Part print with two shaded views. Sizes in mm from the minimum x, y, z corner. Give positions to 0.01 mm unless a question says otherwise; leave off trailing zeros. Order: outer loops, then holes, each group sorted by start corner. A loop starts at its lowest first (then second) coordinate and runs counter-clockwise, first axis right, second up. Notation, with made-up numbers: M 66.25,76 L 87.25,76 A24 cw 87.25,95 Z; hole C 35,48 d8. An arc over 180 degrees is marked long. Answer as CSV lines item,"result".
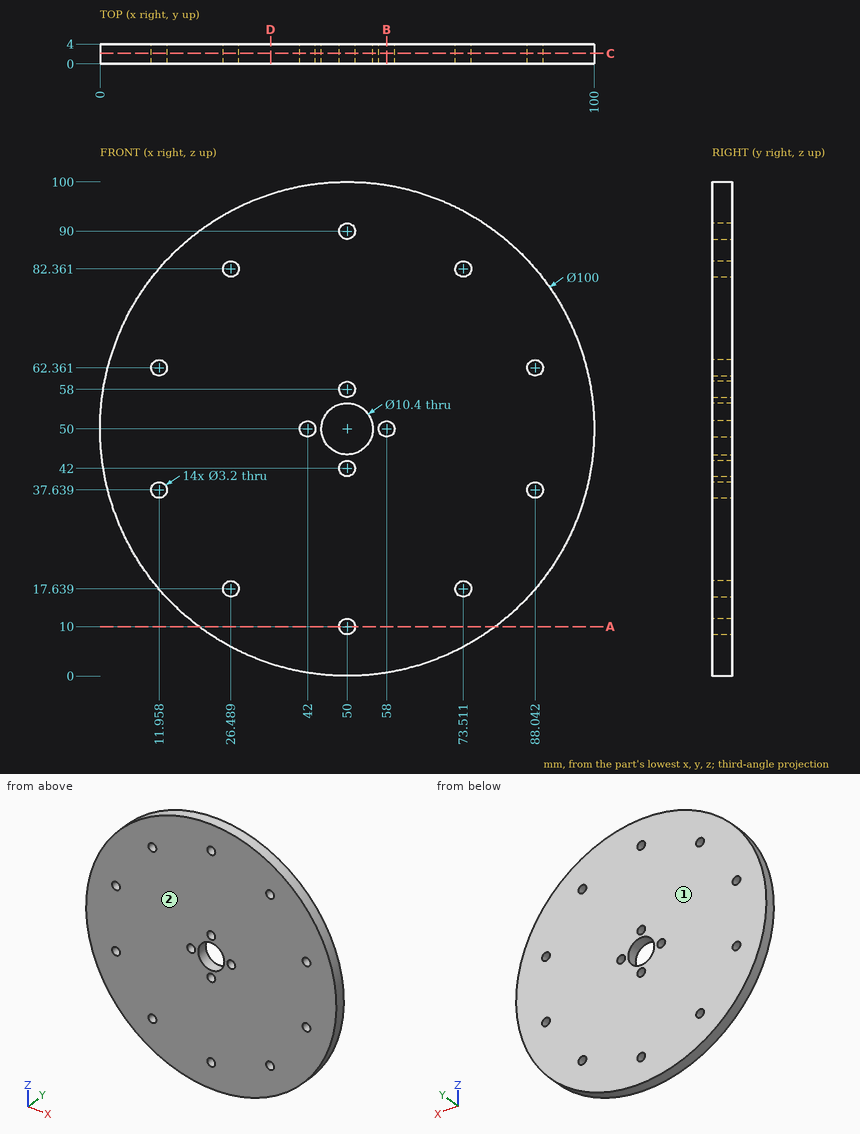
Item 1: Band-saw the part on D-D (x = 34.5). Give the cut face in (y, z), and give its area (3 significant figures).
Geometry says:
outline,"M 0,2.46 L 4,2.46 L 4,97.54 L 0,97.54 Z"
area,"380 mm2"
Item 2: Pull direction Y, two halves, no side cores. Call the marked faces 1 and 2: released by +Y, released by -Y, zero draft, split by the parting line, or undercut.
Geometry says:
face 1,"released by +Y"
face 2,"released by -Y"
Item 3: Band-saw the part on C-C (y = 2.1). State how many separate pieces and enclosed holes the cut face has, and give its area (3 significant figures).
Geometry says:
separate pieces,"1"
enclosed holes,"15"
area,"7,660 mm2"
Item 4: Drop flat-ended pins along their axis: pin 1 (1.5 mm diameter, centred on y = 2.5, z = 59, fed in from -X) (1 decimal); pin 2 (1.9 mm diameter, centred on x = 58, z = 50, fed in from +Y); pin 3 (2 mm diameter, centred on y = 1.5, z = 27.5, fed in from -X); pin 4 (2 mm diameter, centred on y = 1.5, z = 10.5, fed in from +X). Give the stop position or say it passes through.
Geometry says:
pin 1,"stops at x = 0.7"
pin 2,"passes through"
pin 3,"stops at x = 4.86"
pin 4,"stops at x = 81.9"
Item 5: Band-saw the part on A-A (z = 10). Give the cut face in (x, y), and give its area (3 significant figures).
Geometry says:
outline,"M 20,0 L 48.4,0 L 48.4,4 L 20,4 Z; M 51.6,0 L 80,0 L 80,4 L 51.6,4 Z"
area,"227 mm2"
Item 6: Probe line 1 along Z through (x, y) = (87, 0.85) (1 decimal); line 2 along X through (y, z) = (3.05, 18.5); line 3 along Z through (x, y) = (57, 2.6). List the from-to ranges inside material, lowest first. Write a range as from..to.
Geometry says:
line 1,"z = 16.4..36.4, 38.9..61.1, 63.6..83.6"
line 2,"x = 11.17..25.14, 27.84..72.16, 74.86..88.83"
line 3,"z = 0.49..48.75, 51.25..99.51"
Item 7: Band-saw the part on B-B (x = 58). Give the cut face in (y, z), and give its area (3 significant figures).
Geometry says:
outline,"M 0,0.64 L 4,0.64 L 4,48.4 L 0,48.4 Z; M 0,51.6 L 4,51.6 L 4,99.36 L 0,99.36 Z"
area,"382 mm2"
